from build123d import *

# Parameters (mm, degrees)
PAD_DEPTH       = 50
SKETCH001_R     = 23.31
POCKET_DEPTH    = 7
SKETCH002_R     = 2
POCKET001_DEPTH = 7


with BuildPart() as part:
    # Sketch → Pad (new body)
    with BuildSketch(Plane.XZ):
        Polygon((-41.7, -27), (-48.7, -27), (-48.7, 20), (0, 20), (0, 13), (-41.7, 13), align=None)
    extrude(amount=-PAD_DEPTH)

    # Sketch001 → Pocket (cut)
    with BuildSketch(Plane(origin=(0, 0, 20), x_dir=(-1, 0, 0), z_dir=(0, 0, 1))):
        with Locations((-8.31, -25)):
            Circle(SKETCH001_R)
    extrude(amount=-POCKET_DEPTH, mode=Mode.SUBTRACT)

    # Sketch002 → Pocket001 (cut)
    with BuildSketch(Plane(origin=(-48.7, 0, 0), x_dir=(0, 0, -1), z_dir=(-1, 0, 0))):
        with Locations((20, -25)):
            Circle(SKETCH002_R)
    extrude(amount=-POCKET001_DEPTH, mode=Mode.SUBTRACT)


solid = part.part
CAD build for the part. Positions are in the model's coordinates, mm. A direction names the side the tool comes from. Coordinates: 2 decimals unless noted, no trailing zeros. Loops run counter-clockwise (first coordinate to the right, second up) from the corner with the lowest first, then second, coordinate; pieces in that order, holes last. Notation, with made-up numbers: (77.25, 88.25) -> (123.25, 88.25) arc R12 cw to (123.25, 102.25) -> close; hole circle Ø6 at (24, 43). An arc over 180 degrees is marked (long way). One line per item, written item: value.
1. Slice it at B-B on z = -20. Write the cut outline in (x, y).
Answers:
outline: (-48.7, 0) -> (-41.7, 0) -> (-41.7, 23) -> (-48.7, 23) -> close; (-48.7, 27) -> (-41.7, 27) -> (-41.7, 50) -> (-48.7, 50) -> close
2. Which spindle directions (+Z, -Z, +X, -X, +Y, -Y) get a long thin tool onto all of the face, cutting with end or side? Do faces 1 (the face through (-41.7, 25, -7)), 2 (the face through (-35, 50, 14)). Say none if no direction does.
Answers:
face 1: -Z, +X, +Y, -Y
face 2: +Z, -Z, +X, -X, +Y
3. Slice it at C-C on x = -11. Write the cut outline in (y, z), and give its area (3 significant figures).
Answers:
outline: (0, 13) -> (11.94, 13) -> (11.94, 20) -> (0, 20) -> close; (38.06, 13) -> (50, 13) -> (50, 20) -> (38.06, 20) -> close
area: 167 mm^2
4. Drill centre lines: line 1 (Z direction, x = -44, y = 25); line 2 (Y direction, x = -43.75, z = -20); line 3 (X direction, y = 6, z = -6). Where is each one in solid material? Low to high. Write a range as [from, to].
Answers:
line 1: z = [-27, -22], [-18, 20]
line 2: y = [0, 23], [27, 50]
line 3: x = [-48.7, -41.7]
5. Slice it at D-D on z = 16. Write the cut outline in (x, y), and give its area (3 significant figures).
Answers:
outline: (-48.7, 0) -> (0, 0) -> (0, 3.22) arc R23.31 cw to (0, 46.78) -> (0, 50) -> (-48.7, 50) -> close
area: 1,960 mm^2
6. Slice it at A-A on y = 25. Write the cut outline in (x, z).
Answers:
outline: (-48.7, -27) -> (-41.7, -27) -> (-41.7, -22) -> (-48.7, -22) -> close; (-48.7, -18) -> (-41.7, -18) -> (-41.7, 13) -> (-15, 13) -> (-15, 20) -> (-48.7, 20) -> close
7. Flat gauge pins, fed straight in: P1, Ø6, axis at x = -20.5, y = 42.5, coming from the -Z side; P2, Ø4.5, axis at y = 25, z = -20, coming from the -X side; P3, Ø1.5, axis at x = -23.5, z = 11.5, coming from the +Y side; P4, Ø2, axis at y = 9, z = -11, coming from the +X side. Where does each tip first touch, or does it go through?
Answers:
P1: stops at z = 13
P2: stops at x = -48.7
P3: passes through
P4: stops at x = -41.7
8. Pull direction Z, two halves, no side cores. Call faces 3 (the face through (-45.2, 26.2, -18.4)), 4 (the face through (-35, 0, 14)), 5 (the face through (-30, 25, 20)), 6 (the face through (-25, 25, 13)): pulls with the +Z half, pulls with the -Z half, needs draft (parallel to the pull), parting line crosses it, or undercut.
Answers:
face 3: undercut
face 4: needs draft
face 5: pulls with the +Z half
face 6: pulls with the -Z half
